from build123d import *

# Parameters (mm, degrees)
F1_DEPTH      = 19.05
F2_W          = 19.05
F2_H          = 19.05
F3_DEPTH      = 31.75
F3_DEPTH_BACK = 12.7


with BuildPart() as f1:
    # F0 (on Front) → F1 (new body)
    with BuildSketch(Plane.XZ):
        Polygon((1.5262, 48.210221), (0, 0), (101.6, 0), (101.6, 25.4), (53.855859, 25.4), (50.8, 25.4), (39.6262, 48.210221), align=None)
    extrude(amount=F1_DEPTH)

    # F2 (on Front) → F3 (join, two sides)
    with BuildSketch(Plane.XZ) as f3_sk:
        with Locations((9.525, 9.525)):
            Rectangle(F2_W, F2_H)
    extrude(amount=F3_DEPTH)
    extrude(f3_sk.sketch, amount=-F3_DEPTH_BACK)


solid = f1.part
Check sheet for the modelled part. Datum: model origin and axes. Units: mm. A direction names the side the tool comes from. Give positions to 0.01 mm unless a question says otherwise; leave off trailing zeros. Loops run counter-clockwise (first coordinate to the right, second up) from the corner with the lowest first, then second, coordinate; pieces in that order, holes last. Notation, with made-up numbers: M 49.5,18.5 L 75.5,18.5 A15 ccw 75.5,26.5 Z; hole C -18.5,50.25 d8. An arc over 180 degrees is marked long. Answer as a JSON object with one key per item and string values. Group by question number.
Q1. Cross-section at D-D on x = 76. Record the cut outline in (y, z).
Q2. Cross-section at B-B on z = 4. Record the cut outline in (x, y).
Q3. Material ranges on line 1 along Z through (x, y) = (76, -19); line 2 along X through (y, z) = (5.5, 11.5), recorded low to high. Write a range as [from, to].
Q4. Cross-section at A-A on x = 15. Record the cut outline in (y, z).
Q5. Go/stop test with flat-tipped pins: P1, Ø12, axis at y = -2.5, z = 39, coming from the +X side; P2, Ø3, axis at x = 54.5, z = 10, coming from the -Y side; P3, Ø12, axis at x = 64.5, z = 16.5, coming from the +Y side. Record where each tip stops, or that it passes through.
Q6. Access from +Z, -Z, +X, -X, +Y, -Y to the whole of each face (thin tool, end or side, straight path). Record for faces 1 (the flat face through (39, -10, 0)), 2 (the flat face through (19.05, 6, 9)), 3 (the flat face through (77, -9, 25.4)), 4 (the flat face through (19.05, -25, 9)).
Q7. Cross-section at C-C on y = 2.5. Record the cut outline in (x, z).
Evaluation:
{
 "1": {"outline": "M -19.05,0 L 0,0 L 0,25.4 L -19.05,25.4 Z"},
 "2": {"outline": "M 0,-31.75 L 19.05,-31.75 L 19.05,-19.05 L 101.6,-19.05 L 101.6,0 L 19.05,0 L 19.05,12.7 L 0,12.7 Z"},
 "3": {"line 1": "z = [0, 25.4]", "line 2": "x = [0, 19.05]"},
 "4": {"outline": "M -31.75,0 L 12.7,0 L 12.7,19.05 L 0,19.05 L 0,48.21 L -19.05,48.21 L -19.05,19.05 L -31.75,19.05 Z"},
 "5": {"P1": "stops at x = 47.08", "P2": "stops at y = -19.05", "P3": "stops at y = 0"},
 "6": {"face 1": "-Z, +X, -X, +Y, -Y", "face 2": "+Z, -Z, +X, +Y", "face 3": "+Z, +X, +Y, -Y", "face 4": "+Z, -Z, +X, -Y"},
 "7": {"outline": "M 0,0 L 19.05,0 L 19.05,19.05 L 0,19.05 Z"}
}
